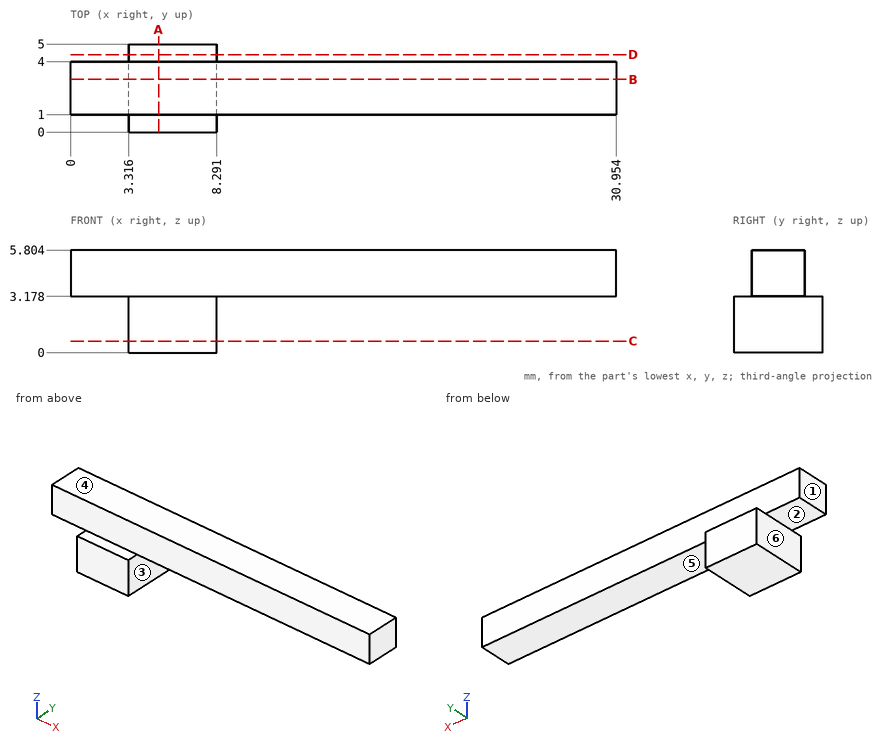
Geometry: see drawing. Coordinates: mm, zero at the bounding-box minimum. A direction names the side the tool comes from. Give positions to 0.01 mm unless a question says otherwise; leave off trailing zeros. Loops run counter-clockwise (first coordinate to the right, second up) from the corner with the lowest first, then second, coordinate; pieces in that order, holes last. Notation, with made-up numbers: (7, 61) -> (34, 61) arc R32 cw to (34, 88) -> close; hole circle Ø10 at (-34, -18.5). An arc over 180 degrees is marked (long way). Use CSV: the item, a comma, the result in double quotes.
(1) Ray query, line 1 along Y through (x, z) = (21, 5.5); line 2 along X through (y, z) = (3.5, 2.4); line 3 along Z through (x, y) = (27, 3.2). Return the intervals inside material, ascending. Write a range as [from, to].
From the geometry:
line 1,"[1, 4]"
line 2,"[3.32, 8.29]"
line 3,"[3.18, 5.8]"
(2) First-contact query: P1, Ø1.6, axis at y = 3, z = 1, coming from the -X side; P2, Ø2, axis at x = 14, z = 5, coming from the +Y side; P3, Ø1.5, axis at x = 16, z = 2.5, coming from the -Y side; P4, Ø2, axis at y = 2, z = 2.5, coming from the -X side. Flat tips, straight axial feed; report the tip coordinate or a pass-through.
From the geometry:
P1,"x = 3.32"
P2,"y = 4"
P3,"y = 1"
P4,"x = 0"
(3) Cut plane A-A (x = 5). Output: boundary loops of the cut face in (y, z).
From the geometry:
outline,"(0, 0) -> (5, 0) -> (5, 3.18) -> (4, 3.18) -> (4, 5.8) -> (1, 5.8) -> (1, 3.18) -> (0, 3.18) -> close"
(4) Pull-direction query (Z, two-part tool) for the marked faces 4, 5 and 6; classes: released by +Z, released by -Z, zero draft, split by the parting line, or undercut.
From the geometry:
face 4,"released by +Z"
face 5,"released by -Z"
face 6,"zero draft"
(5) Access query for the marked faces 1, 2 and 3. Directions: +Z, -Z, +X, -X, +Y, -Y. A direction counts if a zero-diameter tool reaches every point of the face in a straight line with its end or side. Return the directions, or none.
From the geometry:
face 1,"+Z, -Z, -X, +Y, -Y"
face 2,"-Z, -X, +Y, -Y"
face 3,"-Z, +X, +Y, -Y"
(6) Cut plane B-B (y = 3). Output: boundary loops of the cut face in (x, z).
From the geometry:
outline,"(0, 3.18) -> (3.32, 3.18) -> (3.32, 0) -> (8.29, 0) -> (8.29, 3.18) -> (30.95, 3.18) -> (30.95, 5.8) -> (0, 5.8) -> close"
(7) Cut plane C-C (z = 0.65). Output: boundary loops of the cut face in (x, y).
From the geometry:
outline,"(3.32, 0) -> (8.29, 0) -> (8.29, 5) -> (3.32, 5) -> close"
(8) Cut plane D-D (y = 4.4). Output: boundary loops of the cut face in (x, z), plus the area to 3 significant figures.
From the geometry:
outline,"(3.32, 0) -> (8.29, 0) -> (8.29, 3.18) -> (3.32, 3.18) -> close"
area,"15.8 mm^2"
